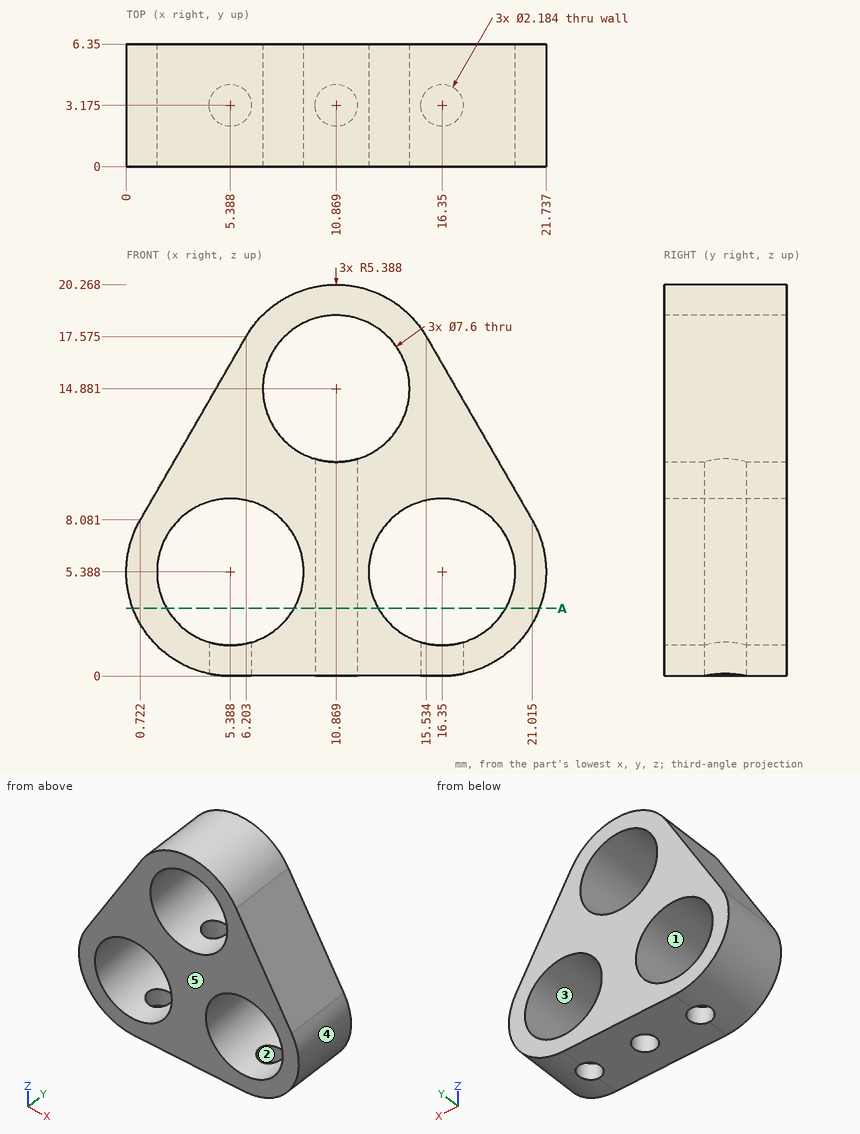
Geometry: see drawing. Coordinates: mm, zero at the bounding-box minimum. A direction names the side the tool comes from. Round coordinates to 2 decimals unless told otherwise and drop trailing zeros.
(1) Pull-direction query (X, two-part tool) for the marked faces 3, 4 and 5; classes: +X half, -X half, draft (parallel to the pull), parting line (faces both ways), or undercut.
From the geometry:
face 3: undercut
face 4: +X half
face 5: draft
(2) Section query A-A (z = 3.5). Give the number of separate pieces and of enclosed holes in the cut face.
From the geometry:
separate pieces: 3
enclosed holes: 1
(3) Contact query for flat-ended pins moving along their axis: pin 1 Ø6 at (x, z) = (5.39, 5.39) entering from -Y; pin 2 Ø2.5 at (x, y) = (5.39, 3.18) entering from -Z; pin 3 Ø1 at (y, z) = (2, 17.5) entering from +X (1 decimal); pin 4 Ø1.5 at (y, z) = (1, 6.5) entering from -X. Output: stop coordinate, or through.
From the geometry:
pin 1: passes through
pin 2: stops at z = 0
pin 3: stops at x = 15.9
pin 4: stops at x = 0.01
(4) Access query for the marked faces 1 and 2. Directions: +Z, -Z, +X, -X, +Y, -Y. A direction counts if a zero-diameter tool reaches every point of the face in a straight line with its end or side. Return the directions, or none.
From the geometry:
face 1: +Y, -Y
face 2: -Z
(5) Material intervals for probe 1 along X at (y, z) = (2, 5.5) (1 decimal); probe 2 along X at (y, z) = (1.75, 8) (1 decimal); probe 3 along Z at (x, y) = (14, 2) (1 decimal), sorted ascending.
From the geometry:
probe 1: x = 0 to 1.6, 9.2 to 12.6, 20.1 to 21.7
probe 2: x = 0.7 to 2.6, 8.1 to 13.6, 19.1 to 21.1
probe 3: z = 0 to 2.4, 8.4 to 12.7, 17 to 19.3
